```python
from build123d import *

# Parameters (mm, degrees)
SKETCH_R     = 17
PAD_DEPTH    = 1
SKETCH001_R  = 13
PAD001_DEPTH = 4.7
SKETCH002_R  = 7.5
PAD002_DEPTH = 3.5
SKETCH003_W  = 31
SKETCH003_H  = 4
PAD003_DEPTH = 1
SKETCH004_R  = 2.75
HOLE_DEPTH   = 9.201


with BuildPart() as part:
    # Sketch → Pad (new body)
    with BuildSketch(Plane.XY):
        Circle(SKETCH_R)
    extrude(amount=PAD_DEPTH)

    # Sketch001 (on Face3 of Pad) → Pad001 (join)
    with BuildSketch(Plane.XY.offset(1)):
        Circle(SKETCH001_R)
    extrude(amount=PAD001_DEPTH)

    # Sketch002 (on Face5 of Pad001) → Pad002 (join)
    with BuildSketch(Plane.XY.offset(5.7)):
        Circle(SKETCH002_R)
    extrude(amount=PAD002_DEPTH)

    # Sketch003 (on Face2 of Pad002) → Pad003 (join)
    with BuildSketch(Plane(origin=(0, 0, 0), x_dir=(1, 0, 0), z_dir=(0, 0, -1))):
        with Locations((15.5, 2)):
            Rectangle(SKETCH003_W, SKETCH003_H)
    extrude(amount=-PAD003_DEPTH)

    # Sketch004 (on Face2 of Pad003) → Hole (cut, through all)
    with BuildSketch(Plane(origin=(0, 0, 0), x_dir=(1, 0, 0), z_dir=(0, 0, -1))):
        Circle(SKETCH004_R)
    extrude(amount=-HOLE_DEPTH, mode=Mode.SUBTRACT)


solid = part.part
```
The listing builds one solid part. Answer for the finished solid, in the listing's coordinates (mm). A direction names the side the tool comes from. Give positions to 0.01 mm unless a question says otherwise; leave off trailing zeros. Loops run counter-clockwise (first coordinate to the right, second up) from the corner with the lowest first, then second, coordinate; pieces in that order, holes last. Notation, with made-up numbers: (52, 46) - (86, 46) arc R30 ccw to (86, 81) - close; hole circle Ø4 at (79.5, -26.75). An arc over 180 degrees is marked (long way). Answer as CSV lines item,"result". Start each with the question number.
Item 1: Find the intervals of material crossed by line 1 (Y direction, x = 0, z = 6.5); line 2 (Y direction, x = 0, z = 4.5); line 3 (Z direction, x = 8.5, y = 11), in increasing order. Write a range as from..to.
Item 2: Each of these flat-tipped pins is pushed along its axis until it touches: pin 1 (1.5 mm diameter, centred on x = 16, z = 3, fed in from +Y); pin 2 (1 mm diameter, centred on x = 19, y = -3, fed in from +Z); pin 3 (1 mm diameter, centred on y = -7, z = 2, fed in from +X); pin 4 (6 mm diameter, centred on x = 10.5, y = 10.5, fed in from +Z). Where does it stop, or does it pass through?
Item 3: A cutting plane is placed at A-A on x = 0. Determine the outline of the cut face in (y, z).
Item 4: For faces 5 (the face through (-7.493, 0.33, 7.426)), 6 (the face through (1, -4, 0)), 7 (the face through (23.9, 0, 0.5)), determine the directions among +Z, -Z, +X, -X, +Y, -Y from which every point of the face is accessible in a straight line to the end or side of a thin tool.
Item 5: A cutting plane is placed at B-B on y = -4.5. Determine the outline of the cut face in (x, z), then the cut area to 3 significant figures.
Item 6: The mould has two halves that part along X. Classify faces 1 (the face through (31, -2, 0.5)), 2 (the face through (-0.596, 2.685, 4.536)), 3 (the face through (23.7, -4, 0.5)), 4 (the face through (-10.316, -7.91, 3.317)): +X half, -X half, draft (parallel to the pull), parting line (faces both ways), or undercut.
Item 7: A cutting plane is placed at C-C on z = 8. Determine the outline of the cut face in (x, y), then the cut area to 3 significant figures.
Item 8: A cutting plane is placed at D-D on x = 16. Determine the outline of the cut face in (y, z), then the cut area to 3 significant figures.
Found:
1,line 1,"y = -7.5..-2.75, 2.75..7.5"
1,line 2,"y = -13..-2.75, 2.75..13"
1,line 3,"z = 0..1"
2,pin 1,"passes through"
2,pin 2,"stops at z = 1"
2,pin 3,"stops at x = 11.26"
2,pin 4,"stops at z = 5.7"
3,outline,"(-17, 0) - (-2.75, 0) - (-2.75, 9.2) - (-7.5, 9.2) - (-7.5, 5.7) - (-13, 5.7) - (-13, 1) - (-17, 1) - close; (2.75, 0) - (17, 0) - (17, 1) - (13, 1) - (13, 5.7) - (7.5, 5.7) - (7.5, 9.2) - (2.75, 9.2) - close"
4,face 5,"+Z"
4,face 6,"-Z, +X, -X, +Y, -Y"
4,face 7,"+Z, -Z, +X, +Y"
5,outline,"(-16.39, 0) - (16.39, 0) - (16.39, 1) - (12.2, 1) - (12.2, 5.7) - (6, 5.7) - (6, 9.2) - (-6, 9.2) - (-6, 5.7) - (-12.2, 5.7) - (-12.2, 1) - (-16.39, 1) - close"
5,area,"189 mm^2"
6,face 1,"+X half"
6,face 2,"undercut"
6,face 3,"draft"
6,face 4,"parting line"
7,outline,"circle Ø15 at (0, 0); hole circle Ø5.5 at (0, 0)"
7,area,"153 mm^2"
8,outline,"(-5.74, 0) - (5.74, 0) - (5.74, 1) - (-5.74, 1) - close"
8,area,"11.5 mm^2"
